Can you work these out from the model? Positions are in its coordinate system, mm. Face numbers are marked on the shaded views. Give positions to 0.01 mm unless a question says otherwise; leave off trailing zeros. Loops run counter-clockwise (first coordinate to the right, second up) from the corner with the lowest first, then second, coordinate; pieces in that order, holes last. Notation, with made-up numbers: M 49,-30.5 L 54,-30.5 A35 cw 54,2.5 Z; hole C 14.5,44.5 d6. An arc over 180 degrees is marked long. Answer as a JSON object with one key per item and string values.
Autodesk Fusion 360 part; units mm, degrees
sketch "Sketch1" plane through (0, 0, 0) normal (0, 0, 1) x (1, 0, 0)
  circle A0 centre (0, 0) radius 15
  circle A1 centre (0, 0) radius 20
  dimension "d1" = 30
  dimension "d2" = 5
extrude "Extrude1" add sketch "Sketch1" along normal blind 21
sketch "Sketch2" plane through (0, 0, 21) normal (0, 0, 1) x (-1, 0, 0)
  circle A0 centre (0, 0) radius 15
  circle A1 centre (0, 0) radius 20
  line L0 (-14.7902, -2.5) -> (-19.8431, -2.5)
  line L1 (-14.7902, 2.5) -> (-19.8431, 2.5)
  line L2 (-14.7902, -2.5) -> (-14.7902, 2.5) construction
  point P0 (-14.7902, 0)
  dimension "d5" = 5
extrude "Extrude2" cut sketch "Sketch2" against normal blind 3 contours A0 A1 L0 L1 picked at (-8.9596, 15.9555)
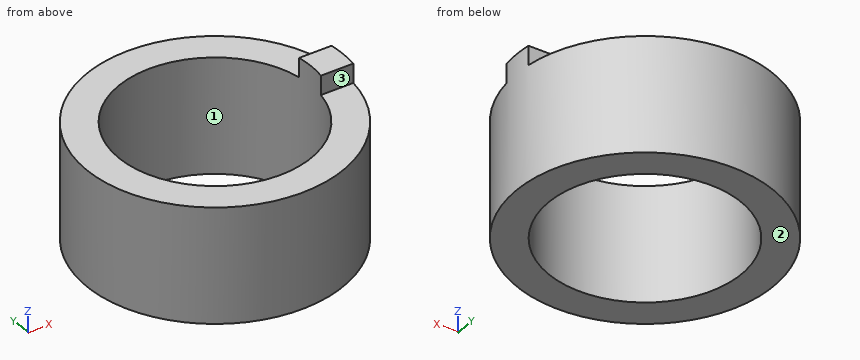
1) Will these pins go through, and if not, where does the flat tip stop? pin 1 Ø0.9 at (x, z) = (18.5, 19) entering from -Y; pin 2 Ø10 at (x, z) = (-13.5, 17.5) entering from +Y; pin 3 Ø3 at (x, z) = (9.5, 10) entering from +Y.
Answer list:
{"pin 1": "y = -2.5", "pin 2": "y = 18.1", "pin 3": "y = 18.33"}
2) If we mould it in two halves opening along Y, with no side actions, what happens to the marked faces 1, 2 and 3? For each: +Y half, -Y half, draft (parallel to the pull), parting line (faces both ways), or undercut.
Answer list:
{"face 1": "undercut", "face 2": "draft", "face 3": "-Y half"}
3) Suppose I cut it at B-B, the plane x = 0. Write out the boundary of the cut face in (y, z).
Answer list:
{"outline": "M -20,0 L -15,0 L -15,18 L -20,18 Z; M 15,0 L 20,0 L 20,18 L 15,18 Z"}
4) Suppose I cut it at D-D, the plane z = 19.25. Write out the boundary of the cut face in (x, y).
Answer list:
{"outline": "M 14.79,-2.5 L 19.84,-2.5 A20 ccw 19.84,2.5 L 14.79,2.5 A15 cw Z"}
5) Suppose I cut it at C-C, the plane z = 13.5. Write out the boundary of the cut face in (x, y), and give its area (3 significant figures).
Answer list:
{"outline": "C 0,0 d40; hole C 0,0 d30", "area": "550 mm^2"}
6) Please list where these lines run through material, in increasing order: line 1 along Y through (x, z) = (0, 6.75); line 2 along Z through (x, y) = (11, 15). Write a range as from..to.
Answer list:
{"line 1": "-20..-15, 15..20", "line 2": "0..18"}
7) Suppose I cut it at A-A, the plane y = 0. Write out the boundary of the cut face in (x, z).
Answer list:
{"outline": "M -20,0 L -15,0 L -15,18 L -20,18 Z; M 15,0 L 20,0 L 20,21 L 15,21 Z"}
